Could you check a few things on this drawing? It's one solid part, dimensions in mm from its lowest x, y, z. Give positions to 0.01 mm unless a question says otherwise; leave off trailing zeros. Order: outer loops, then holes, each group sorted by start corner. A loop starts at its lowest first (then second) coordinate and runs counter-clockwise, first axis right, second up.
Item 1: I want a section at C-C, the plane x = 153. Write out the boundary of the cut face in (y, z) (1 decimal).
Item 2: If I drill on line 1 along X through (y, z) = (62.5, 1.8); line 2 along X through (y, z) = (7, 1.25); line 3 along X through (y, z) = (65, 2.55), over which ranges is the centre line in solid material (lowest first)?
Item 3: I'm going to push flat-ended pins straight in: pin 1 Ø1 at (x, z) = (150, 1) entering from +Y; pin 2 Ø1 at (x, z) = (152, 1) entering from +Y. Where does each tip first touch, or does it pass through?
Item 4: I want a section at B-B, the plane z = 0.6. Count the separate pieces of the cut face and the enclosed holes in it, then the cut area to 3 significant figures.
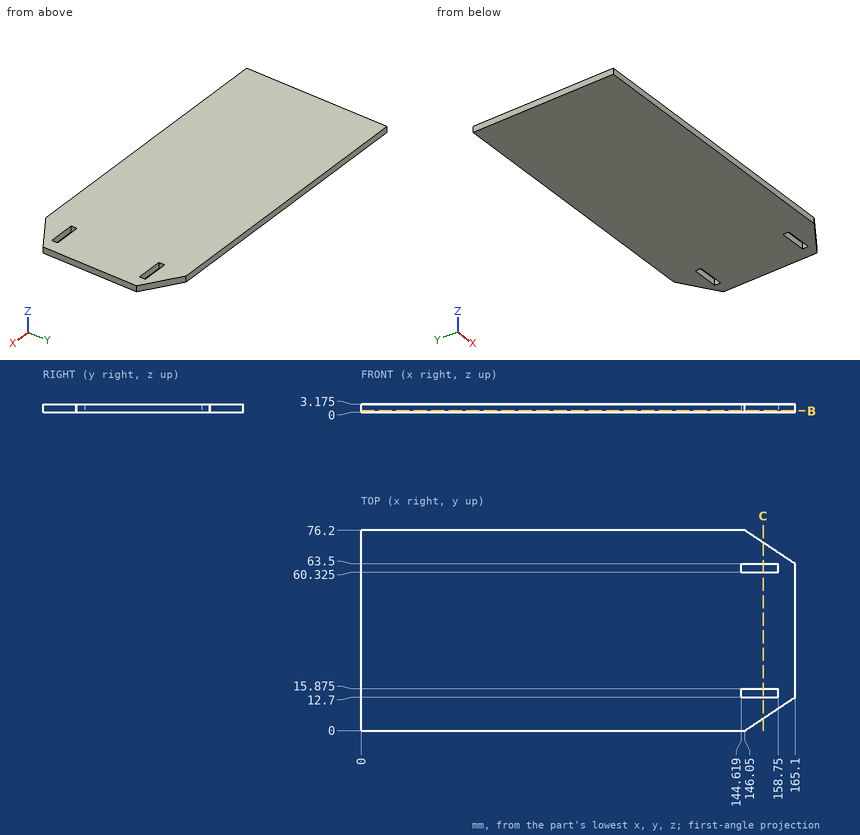
Results list:
1. outline: (4.6, 0) - (12.7, 0) - (12.7, 3.2) - (4.6, 3.2) - close; (15.9, 0) - (60.3, 0) - (60.3, 3.2) - (15.9, 3.2) - close; (63.5, 0) - (71.6, 0) - (71.6, 3.2) - (63.5, 3.2) - close
2. line 1: x = 0 to 144.62, 158.75 to 165.1
2. line 2: x = 0 to 156.55
2. line 3: x = 0 to 162.85
3. pin 1: stops at y = 73.9
3. pin 2: stops at y = 72.57
4. separate pieces: 1
4. enclosed holes: 2
4. area: 12,200 mm2
